Geometry check sheet. Reference: the model listing, model coordinates, mm. Face numbers are marked on the shaded views. Give positions to 0.01 mm unless a question says otherwise; leave off trailing zeros. Write each loop counter-clockwise with the first axis right and the second up, starting at its lowest first coordinate (ties: lowest second). Pieces come first, ordered by that corner, then holes. Notation, with made-up numbers: (41.25, 70) - (89.25, 70) arc R7 ccw to (89.25, 83) - close; hole circle Ø8 at (-31.75, 69.5). An arc over 180 degrees is marked (long way). One line per question, with ' | ' between items. Start each with the question number.
Q1. Section check A-A on y = 12.5. Count the separate pieces of the cut face and the enclosed holes in it, and give its area (3 significant figures).
Q2. Section check D-D on x = -8.25. Record the boundary of the cut face in (y, z).
Q3. Gauge pin test, flat ends, axial feed: P1, Ø4, axis at x = 7, z = 10.5, coming from the -Y side; P2, Ø1.5, axis at x = -4, z = 4.5, coming from the +Y side; P3, Ø2, axis at x = -10, z = -10, coming from the +Y side; P4, Ø3, axis at x = 13, z = -9, coming from the +Y side. Record the tip position at first contact, or that the pin passes through.
Q4. Release check for a two-part mould opening along X. For the marked faces 1, 2 and 3 record: +X half, -X half, draft (parallel to the pull), parting line (faces both ways), or undercut.
Q5. Section check B-B on x = 0. Record the boundary of the cut face in (y, z).
Q6. Section check C-C on z = 7. Record the boundary of the cut face in (x, y).
Q7. Thickness scan on L1, parallel to Z at x = 13, y = 13.7; L2, parallel to Z at x = -10, y = 13; L3, parallel to X at y = 12.75, z = 10. Record the ranges inside material, lowest first. Write a range as [from, to].
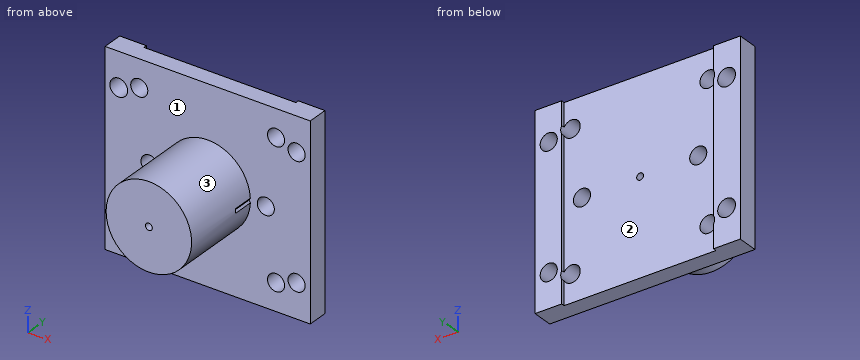
Autodesk Inventor part; units mm, degrees
ref_plane "YZ Plane" through (0, 0, 0) normal (1, 0, 0) x (0, 1, 0)
ref_plane "XZ Plane" through (0, 0, 0) normal (0, 1, 0) x (-1, 0, 0)
ref_plane "XY Plane" through (0, 0, 0) normal (0, 0, 1) x (1, 0, 0)
sketch "Sketch1" plane through (0, 0, 0) normal (0, 1, 0) x (-1, 0, 0)
  circle A0 centre (0, 0) radius 6.25
  dimension "d0" = 12.5
extrude "Extrusion1" add sketch "Sketch1" along normal blind 12
sketch "Sketch2" plane through (0, 12, 0) normal (0, 1, 0) x (1, 0, 0)
  line L0 (-15, 14) -> (15, 14)
  line L1 (15, 14) -> (15, -14)
  line L2 (15, -14) -> (-15, -14)
  line L3 (-15, -14) -> (-15, 14)
  point P0 (0, 0)
  dimension "d3" = 30
  dimension "d4" = 28
  dimension "d5" = 14
  dimension "d6" = 15
extrude "Extrusion2" add sketch "Sketch2" along normal blind 3
sketch "Sketch3" plane through (0, 15, 0) normal (0, 1, 0) x (1, 0, 0)
  line L0 (-15, -14) -> (15, -14)
  line L1 (15, 14) -> (-15, 14)
  line L2 (11.1, -14) -> (-11.1, -14)
  line L3 (-11.1, -14) -> (-11.1, 14)
  line L4 (-11.1, 14) -> (11.1, 14)
  line L5 (11.1, 14) -> (11.1, -14)
  line L6 (-15, 14) -> (-15, -14)
  point P0 (0, 0)
  point P1 (11.1, 14)
  point P2 (-11.1, -14)
  dimension "d9" = 22.2
  dimension "d10" = 3.9
extrude "Extrusion3" cut sketch "Sketch3" against normal blind 0.5 contours L3 L1 L5 L0
sketch "Sketch4" plane through (0, 14.5, 0) normal (0, 1, 0) x (1, 0, 0)
  circle A0 centre (8.5, 0) radius 1.25
  circle A1 centre (-8.5, 0) radius 1.25
  point P0 (0, 0)
  dimension "d13" = 2.5
  dimension "d14" = 8.5
  dimension "d15" = 2.5
  dimension "d16" = 8.5
extrude "Extrusion4" cut sketch "Sketch4" against normal blind 5
sketch "Sketch5" plane through (0, 12, 0) normal (0, -1, 0) x (1, 0, 0)
  line L0 (7.4961, 2.1) -> (15, 2.1)
  line L1 (15, 2.1) -> (15, -2.1)
  line L2 (15, -2.1) -> (7.4961, -2.1)
  line L3 (7.4961, -2.1) -> (7.4961, 2.1)
  line L4 (15, 14) -> (15, -14)
  circle A0 centre (8.5, 0) radius 1.25
  line L5 (9.75, 2.1) -> (10.9437, -0.0325)
  line L6 (10.9437, -0.0325) -> (9.6937, -2.1325)
  line L7 (9.6937, -2.1325) -> (7.25, -2.1)
  line L8 (7.25, -2.1) -> (6.0563, 0.0325)
  line L9 (6.0563, 0.0325) -> (7.3063, 2.1325)
  line L10 (7.3063, 2.1325) -> (9.75, 2.1)
  line L11 (-15, -14) -> (-15, 14)
  line L12 (-15, -2.1) -> (-7.25, -2.1)
  line L13 (-7.25, -2.1) -> (-7.25, 2.1)
  line L14 (-7.25, 2.1) -> (-15, 2.1)
  line L15 (-15, 2.1) -> (-15, -2.1)
  circle A1 centre (-8.5, 0) radius 1.25
  line L16 (-7.25, 2.1) -> (-6.0563, -0.0325)
  line L17 (-6.0563, -0.0325) -> (-7.3063, -2.1325)
  line L18 (-7.3063, -2.1325) -> (-9.75, -2.1)
  line L19 (-9.75, -2.1) -> (-10.9437, 0.0325)
  line L20 (-10.9437, 0.0325) -> (-9.6937, 2.1325)
  line L21 (-9.6937, 2.1325) -> (-7.25, 2.1)
  point P0 (0, 0)
  point P1 (9.713, -2.1)
  point P2 (-9.713, 2.1)
  dimension "d19" = 4.2
  dimension "d20" = 0
  dimension "d21" = 2.1
  dimension "d24" = 4.2
  dimension "d25" = 2.1
extrude "Extrusion5" cut sketch "Sketch5" along normal blind 3 contours L3 A0 L2 L6 L7 L8 L9 L10 L0 | L0 L5 L6 L2 L3 A0 | L0 L1 L2 L6 L5 | A0 L3 | L3 A0 | L11 L14 L20 L19 L12 | A1 | L19 L20 L14 L13 L17 L12 | L12 L17 L18 | L20 L21 L14 | L16 L17 L13
sketch "Sketch6" plane through (0, 14.5, 0) normal (0, 1, 0) x (1, 0, 0)
  line L0 (-11.1, -14) -> (-11.1, 14)
  line L1 (-11.1, 11) -> (11.1, 11)
  line L2 (11.1, 11) -> (11.1, -11)
  line L3 (11.1, -11) -> (-11.1, -11)
  line L4 (-11.1, -11) -> (-11.1, 11)
  line L5 (-11.1, 14) -> (11.1, 14)
  circle A0 centre (-13, -9) radius 1.3
  line L6 (-15, -14) -> (-11.1, -14)
  circle A1 centre (-13, 9) radius 1.3
  line L7 (-11.1, 14) -> (-15, 14)
  circle A2 centre (13, 9) radius 1.25
  line L8 (11.1, 14) -> (11.1, -14)
  circle A3 centre (13, -9) radius 1.25
  line L9 (11.1, -14) -> (15, -14)
  point P0 (0, 0)
  dimension "d26" = 22.2
  dimension "d27" = 22
  dimension "d28" = 3
  dimension "d29" = 2.6
  dimension "d30" = 1.9
  dimension "d31" = 5
  dimension "d32" = 2.6
  dimension "d33" = 1.9
  dimension "d34" = 5
  dimension "d35" = 2.5
  dimension "d36" = 1.9
  dimension "d37" = 5
  dimension "d38" = 2.5
  dimension "d39" = 1.9
  dimension "d40" = 5
extrude "Extrusion6" cut sketch "Sketch6" along normal mid plane 5 contours A0 | A1 | A2 | A3
sketch "Sketch7" plane through (0, 14.5, 0) normal (0, 1, 0) x (1, 0, 0)
  circle A0 centre (-10, 10) radius 1.25
  line L0 (0, 0) -> (4.1718, 0)
  line L1 (0, 0) -> (0, 4.2645)
  circle A1 centre (10, 10) radius 1.25
  circle A2 centre (-10, -10) radius 1.25
  circle A3 centre (10, -10) radius 1.25
  dimension "d43" = 2.5
  dimension "d44" = 10
  dimension "d45" = 10
  dimension "d48" = 20
  dimension "d51" = 20
extrude "Extrusion7" cut sketch "Sketch7" along normal blind 10 and the other way blind 5
sketch "Sketch8" plane through (0, 12, 0) normal (0, -1, 0) x (1, 0, 0)
  arc A0 (11.1, -9.4063) -> (11.1, -10.5937) centre (10, -10) ccw
  circle A1 centre (10, -10) radius 2.5
  circle A2 centre (-10, -10) radius 1.25
  circle A3 centre (-10, -10) radius 2.5
  arc A4 (-11.1, 9.4063) -> (-11.1, 10.5937) centre (-10, 10) ccw
  circle A5 centre (-10, 10) radius 2.5
  arc A6 (11.1, 10.5937) -> (11.1, 9.4063) centre (10, 10) ccw
  circle A7 centre (10, 10) radius 2.5
  point P0 (0, 0)
  dimension "d58" = 5
  dimension "d59" = 5
  dimension "d60" = 5
  dimension "d61" = 5
extrude "Extrusion8" cut sketch "Sketch8" along normal blind 5
sketch "Sketch9" plane through (0, 14.5, 0) normal (0, 1, 0) x (1, 0, 0)
  point P0 (0, 0)
  point P1 (0, 0)
hole "Hole1" at (0, 14.5, 0) direction (0, -1, 0) diameter 1 end through all
properties part number "200205 - Holder for MEMS on halfinch mount"
Working result:
1) separate pieces: 1 | enclosed holes: 11 | area: 789 mm2
2) outline: (12, -14) - (14.5, -14) - (14.5, -1.22) - (12, -1.22) - close; (12, 1.22) - (14.5, 1.22) - (14.5, 14) - (12, 14) - close
3) P1: stops at y = 12 | P2: stops at y = 14.5 | P3: passes through | P4: stops at y = 15
4) face 1: draft | face 2: undercut | face 3: parting line
5) outline: (0, -6.25) - (12, -6.25) - (12, -14) - (14.5, -14) - (14.5, -0.5) - (0, -0.5) - close; (0, 0.5) - (14.5, 0.5) - (14.5, 14) - (12, 14) - (12, 6.25) - (0, 6.25) - close
6) outline: (-15, 12) - (15, 12) - (15, 15) - (11.1, 15) - (11.1, 14.5) - (-11.1, 14.5) - (-11.1, 15) - (-15, 15) - close
7) L1: z = [-14, -10.25], [-7.75, 7.75], [10.25, 14] | L2: z = [-14, -11.25], [-8.75, 8.75], [11.25, 14] | L3: x = [-15, -13.83], [-12.17, -11.25], [-8.75, 8.75], [11.25, 12.25], [13.75, 15]
